Geometry check sheet. Reference: the model listing, model coordinates, mm. Face numbers are marked on the shaded views. A direction names the side the tool comes from. Give positions to 0.01 mm unless a question says otherwise; leave off trailing zeros. Loops run counter-clockwise (first coordinate to the right, second up) from the corner with the lowest first, then second, coordinate; pieces in that order, holes last.
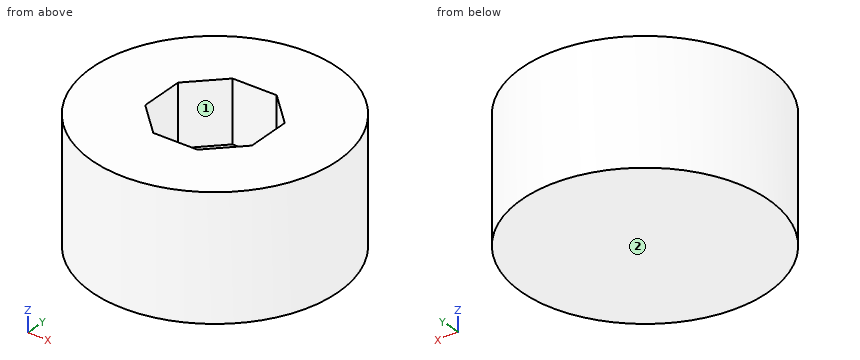
```python
from build123d import *

# Parameters (mm, degrees)
F0_R     = 50
F1_DEPTH = 50
F3_DEPTH = 25


with BuildPart() as f1:
    # F0 (on Top) → F1 (new body)
    with BuildSketch(Plane.XY):
        Circle(F0_R)
    extrude(amount=F1_DEPTH)

    # F2 (on face) → F3 (cut)
    with BuildSketch(Plane.XY.offset(50)):
        Polygon((-8.982444, -21.685537), (8.982444, -21.685537), (21.685537, -8.982444), (21.685537, 8.982444), (8.982444, 21.685537), (-8.982444, 21.685537), (-21.685537, 8.982444), (-21.685537, -8.982444), align=None)
    extrude(amount=-F3_DEPTH, mode=Mode.SUBTRACT)


solid = f1.part
```
1) Scan lines: line 1 along X through (y, z) = (1.5, 34); line 2 along Z through (x, y) = (-0.5, -1.5); line 3 along X through (y, z) = (-4, 47.5). Record each from-to range of solid material in increasing order.
2) Depth check by flat-ended pin: P1, Ø12, axis at y = -34, z = 44.5, coming from the +X side; P2, Ø4, axis at y = 17.5, z = 34.5, coming from the -X side; P3, Ø10, axis at y = -18.5, z = 7.5, coming from the -X side. Enter the tip coordinate at first touch or a pass-through.
3) Sectioned sample at A-A on x = 0. Enter the section's corners in (y, z), plus the area to 3 significant figures.
4) Sectioned sample at D-D on z = 18. Enter the section's corners in (x, y).
5) Tool access check on the marked faces 1 and 2. Record the directions out of +Z, -Z, +X, -X, +Y, -Y that give a thin tool (end or side, any length) a straight path to the whole face; none if there is none.
6) Sectioned sample at B-B on z = 31. Enter the section's corners in (x, y).
Determined:
1. line 1: x = -49.98 to -21.69, 21.69 to 49.98
1. line 2: z = 0 to 25
1. line 3: x = -49.84 to -21.69, 21.69 to 49.84
2. P1: stops at x = 41.42
2. P2: stops at x = -47.54
2. P3: stops at x = -48.14
3. outline: (-50, 0) - (50, 0) - (50, 50) - (21.69, 50) - (21.69, 25) - (-21.69, 25) - (-21.69, 50) - (-50, 50) - close
3. area: 3,920 mm2
4. outline: circle Ø100 at (0, 0)
5. face 1: +Z
5. face 2: -Z, +X, -X, +Y, -Y
6. outline: circle Ø100 at (0, 0); hole (-21.69, -8.98) - (-8.98, -21.69) - (8.98, -21.69) - (21.69, -8.98) - (21.69, 8.98) - (8.98, 21.69) - (-8.98, 21.69) - (-21.69, 8.98) - close
